Input: part model. Units: mm. Frame: model coordinates. Face numbers are marked on the shaded views. A direction names the side the tool comes from. Round coordinates to 2 decimals unless told otherwise and drop trailing zeros. Write each loop counter-clockwise with the first axis right and the second up, starting at its lowest first coordinate (ties: lowest second). Pieces come first, ordered by that corner, then holes. Notation, with made-up numbers: M -28,-8.75 L -20,-8.75 A21 cw -20,26.25 Z; hole C 40.5,12 d5. An arc over 180 degrees is marked long. Answer as CSV lines item,"result". Start each with the question number.
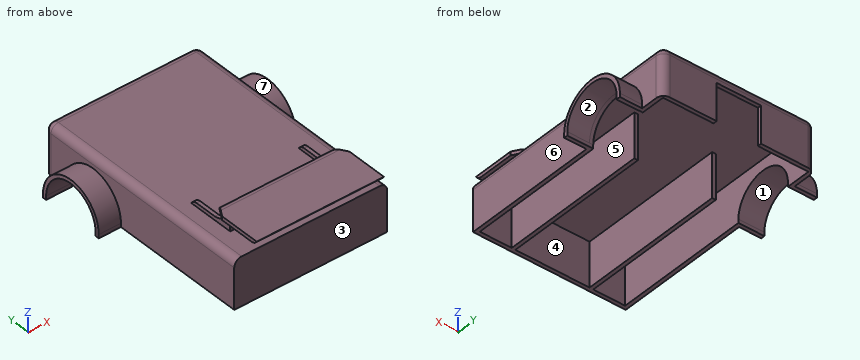
```python
from build123d import *

# Parameters (mm, degrees)
SKETCH1_W               = 206
SKETCH1_H               = 306
BOSS_EXTRUDE2_DEPTH     = 5
SKETCH2_W               = 206
SKETCH2_H               = 306
SKETCH2_W_2             = 196
SKETCH2_H_2             = 296
BOSS_EXTRUDE3_DEPTH     = 60
SKETCH3_W               = 5
SKETCH3_H               = 198
BOSS_EXTRUDE4_DEPTH     = 60
SKETCH10_W              = 60
SKETCH10_H              = 5
CUT_EXTRUDE3_DEPTH      = 50
CUT_EXTRUDE4_DEPTH      = 296.372645991
CUT_EXTRUDE4_DEPTH_BACK = 5
BOSS_EXTRUDE6_DEPTH     = 30
CUT_EXTRUDE5_DEPTH      = 318.025235589
CUT_EXTRUDE5_DEPTH_BACK = 5
BOSS_EXTRUDE7_DEPTH     = 30
SKETCH16_W              = 5
SKETCH16_H              = 63
BOSS_EXTRUDE8_DEPTH     = 5
BOSS_EXTRUDE10_DEPTH    = 150
SKETCH19_W              = 140
SKETCH19_H              = 20
CUT_EXTRUDE6_DEPTH      = 70
BOSS_EXTRUDE11_DEPTH    = 5
FILLET3_R               = 10
FILLET4_R               = 10
FILLET5_R               = 10
FILLET6_R               = 10
FILLET7_R               = 10
FILLET8_R               = 10
FILLET9_R               = 10


with BuildPart() as part:
    # Sketch1 → Boss-Extrude2 (new body)
    with BuildSketch(Plane.XY):
        with Locations((0, 50)):
            Rectangle(SKETCH1_W, SKETCH1_H)
    extrude(amount=BOSS_EXTRUDE2_DEPTH)

    # Sketch2 → Boss-Extrude3 (add)
    with BuildSketch(Plane(origin=(0, 0, 0), x_dir=(-1, 0, 0), z_dir=(0, 0, -1))):
        with Locations((0, 50)):
            Rectangle(SKETCH2_W, SKETCH2_H)
        with Locations((0, 50)):
            Rectangle(SKETCH2_W_2, SKETCH2_H_2, mode=Mode.SUBTRACT)
    extrude(amount=BOSS_EXTRUDE3_DEPTH)

    # Sketch3 → Boss-Extrude4 (add)
    with BuildSketch(Plane(origin=(0, 0, 0), x_dir=(-1, 0, 0), z_dir=(0, 0, -1))):
        with Locations((-52.5, 1)):
            Rectangle(SKETCH3_W, SKETCH3_H)
        with Locations((52.5, 1)):
            Rectangle(SKETCH3_W, SKETCH3_H)
    extrude(amount=BOSS_EXTRUDE4_DEPTH)

    # Sketch10 → Cut-Extrude3 (cut)
    with BuildSketch(Plane(origin=(0, 0, -60), x_dir=(-1, 0, 0), z_dir=(0, 0, -1))):
        with Locations((0, 200.5)):
            Rectangle(SKETCH10_W, SKETCH10_H)
    extrude(amount=-CUT_EXTRUDE3_DEPTH, mode=Mode.SUBTRACT)

    # Sketch11 → Cut-Extrude4 (cut, two sides: drawn at the far end of the back side and taken through both)
    with BuildSketch(Plane(origin=(103, 0, 0), x_dir=(0, 0, -1), z_dir=(1, 0, 0)).offset(-CUT_EXTRUDE4_DEPTH_BACK)):
        with BuildLine():
            Line((55, 165.246993189), (60, 165.246993189))
            Line((60, 165.246993189), (60, 85.246993189))
            Line((60, 85.246993189), (55, 85.246993189))
            ThreePointArc((55, 85.246993189), (15, 125.246993189), (55, 165.246993189))
        make_face()
    extrude(amount=CUT_EXTRUDE4_DEPTH + CUT_EXTRUDE4_DEPTH_BACK, mode=Mode.SUBTRACT)

    # Sketch12 → Boss-Extrude6 (add)
    with BuildSketch(Plane(origin=(103, 0, 0), x_dir=(0, 0, -1), z_dir=(1, 0, 0))):
        with BuildLine():
            Line((55, 170.246993189), (60, 170.246993189))
            Line((60, 170.246993189), (60, 164.922358247))
            Line((60, 164.922358247), (55, 164.922358247))
            ThreePointArc((55, 164.922358247), (15.162317471, 125.084675718), (55, 85.246993189))
            Line((55, 85.246993189), (60, 85.246993189))
            Line((60, 85.246993189), (60, 80.246993189))
            Line((60, 80.246993189), (55, 80.246993189))
            ThreePointArc((55, 80.246993189), (10, 125.246993189), (55, 170.246993189))
        make_face()
    extrude(amount=BOSS_EXTRUDE6_DEPTH)

    # Sketch13 → Cut-Extrude5 (cut, two sides: drawn at the far end of the back side and taken through both)
    with BuildSketch(Plane.ZY.offset(103).offset(-CUT_EXTRUDE5_DEPTH_BACK)):
        with BuildLine():
            Line((-55, 165), (-60, 165))
            Line((-60, 165), (-60, 85))
            Line((-60, 85), (-55, 85))
            ThreePointArc((-55, 85), (-15, 125), (-55, 165))
        make_face()
    extrude(amount=CUT_EXTRUDE5_DEPTH + CUT_EXTRUDE5_DEPTH_BACK, mode=Mode.SUBTRACT)

    # Sketch14 → Boss-Extrude7 (add)
    with BuildSketch(Plane.ZY.offset(103)):
        with BuildLine():
            Line((-55, 170), (-60, 170))
            Line((-60, 170), (-60, 165))
            Line((-60, 165), (-55, 165))
            ThreePointArc((-55, 165), (-15, 125), (-55, 85))
            Line((-55, 85), (-60, 85))
            Line((-60, 85), (-60, 80))
            Line((-60, 80), (-55, 80))
            ThreePointArc((-55, 80), (-10, 125), (-55, 170))
        make_face()
    extrude(amount=BOSS_EXTRUDE7_DEPTH)

    # Sketch16 → Boss-Extrude8 (add)
    with BuildSketch(Plane.XY.offset(5)):
        with Locations((-72.5, -31.5)):
            Rectangle(SKETCH16_W, SKETCH16_H)
        with Locations((72.5, -31.5)):
            Rectangle(SKETCH16_W, SKETCH16_H)
    extrude(amount=BOSS_EXTRUDE8_DEPTH)

    # Sketch17 → Boss-Extrude10 (add)
    with BuildSketch(Plane.ZY.offset(75)):
        with BuildLine():
            Line((5, -63), (30, -63))
            Line((30, -63), (30, -57.184020249))
            ThreePointArc((30, -57.184020249), (16.143353283, -51.612696786), (10, -38))
            Line((10, -38), (10, 0))
            Line((10, 0), (5, 0))
            Line((5, 0), (5, -63))
        make_face()
    extrude(amount=-BOSS_EXTRUDE10_DEPTH)

    # Sketch19 → Cut-Extrude6 (cut)
    with BuildSketch(Plane.XZ.offset(63)):
        with Locations((0, 15)):
            Rectangle(SKETCH19_W, SKETCH19_H)
    extrude(amount=-CUT_EXTRUDE6_DEPTH, mode=Mode.SUBTRACT)

    # Sketch20 → Boss-Extrude11 (add)
    with BuildSketch(Plane.XY.offset(30)):
        Polygon((75, -45.439640401), (-75, -45.439640401), (-85.792774028, -63), (-85.792774028, -118.716663175), (85.792774028, -118.716663175), (85.792774028, -63), align=None)
    extrude(amount=-BOSS_EXTRUDE11_DEPTH)

    # Fillet3
    fillet3_edges = [part.edges().sort_by_distance(p)[0] for p in [
        (-103, 203, -27.5),
    ]]
    fillet(fillet3_edges, radius=FILLET3_R)

    # Fillet4
    fillet4_edges = [part.edges().sort_by_distance(p)[0] for p in [
        (103, 203, -27.5),
    ]]
    fillet(fillet4_edges, radius=FILLET4_R)

    # Fillet5
    # the kernel refuses this fillet: 10 mm, written as the material it takes off along each edge
    with BuildSketch(Plane(origin=(96.650635095, -45.439640401, 30), x_dir=(0, 0, -1), z_dir=(-1, 0, 0))) as fillet5_piece_1:
        with BuildLine():
            CenterArc((10, 8.660254038), FILLET5_R, 180, 60)
            Line((0, 8.660254038), (-0.2, 8.660254038))
            Line((-0.2, 8.660254038), (-0.2, 0))
            Line((-0.2, 0), (0, -0.2))
            ThreePointArc((0, -0.2), (2.5, -0.2), (4.9, -0.173205081))
            Line((4.9, -0.173205081), (5, 0))
        make_face()
    extrude(amount=193.301270189, mode=Mode.SUBTRACT)

    # Fillet6
    # the kernel refuses this fillet: 10 mm, written as the material it takes off along each edge
    with BuildSketch(Plane(origin=(-107.443409123, -118.716663175, 25), x_dir=(0, 1, 0), z_dir=(1, 0, 0))) as fillet6_piece_1:
        with BuildLine():
            CenterArc((8.660254038, 10), FILLET6_R, 210, 60)
            Line((0, 5), (-0.173205081, 4.9))
            ThreePointArc((-0.173205081, 4.9), (-0.2, 2.5), (-0.2, 0))
            Line((-0.2, 0), (0, -0.2))
            Line((0, -0.2), (8.660254038, -0.2))
            Line((8.660254038, -0.2), (8.660254038, 0))
        make_face()
    extrude(amount=214.886818246, mode=Mode.SUBTRACT)

    # Fillet7
    # the kernel refuses this fillet: 10 mm, written as the material it takes off along each edge
    with BuildSketch(Plane(origin=(-96.650635095, 0, 10), x_dir=(0, 0, -1), z_dir=(1, 0, 0))) as fillet7_piece_1:
        with BuildLine():
            CenterArc((10, -8.660254038), FILLET7_R, 120, 60)
            Line((0, -8.660254038), (-0.2, -8.660254038))
            Line((-0.2, -8.660254038), (-0.2, 0))
            Line((-0.2, 0), (0, 0.2))
            ThreePointArc((0, 0.2), (2.5, 0.2), (4.9, 0.173205081))
            Line((4.9, 0.173205081), (5, 0))
        make_face()
    extrude(amount=48.301270189, mode=Mode.SUBTRACT)

    # Fillet8
    # the kernel refuses this fillet: 10 mm, written as the material it takes off along each edge
    with BuildSketch(Plane(origin=(48.349364905, 0, 10), x_dir=(0, 0, -1), z_dir=(1, 0, 0))) as fillet8_piece_1:
        with BuildLine():
            CenterArc((10, -8.660254038), FILLET8_R, 120, 60)
            Line((0, -8.660254038), (-0.2, -8.660254038))
            Line((-0.2, -8.660254038), (-0.2, 0))
            Line((-0.2, 0), (0, 0.2))
            ThreePointArc((0, 0.2), (2.5, 0.2), (4.9, 0.173205081))
            Line((4.9, 0.173205081), (5, 0))
        make_face()
    extrude(amount=48.301270189, mode=Mode.SUBTRACT)

    # Fillet9
    # the kernel refuses this fillet: 10 mm, written as the material it takes off along each edge
    with BuildSketch(Plane(origin=(103, 193, 5), x_dir=(-1, 0, 0), z_dir=(0, -1, 0)), Plane(origin=(-103, -128, 5), x_dir=(1, 0, 0), z_dir=(0, 1, 0))) as fillet9_piece_1:
        with BuildLine():
            CenterArc((FILLET9_R, FILLET9_R), FILLET9_R, 180, 90)
            Line((0, FILLET9_R), (0, 0))
            Line((0, 0), (FILLET9_R, 0))
        make_face()
    extrude(amount=321, mode=Mode.SUBTRACT)
    with BuildSketch(Plane(origin=(-93, 193, 5), x_dir=(-1, 0, 0), z_dir=(0, -1, 0))) as fillet9_piece_2:
        with BuildLine():
            CenterArc((10 - FILLET9_R, FILLET9_R), FILLET9_R, 270, 90)
            Line((10, FILLET9_R), (10, 0))
            Line((10, 0), (10 - FILLET9_R, 0))
        make_face()
    revolve(axis=Axis((-93, 193, 5), (0, 0, -1)), revolution_arc=90, mode=Mode.SUBTRACT)
    with BuildSketch(Plane(origin=(-93, 203, 5), x_dir=(0, -1, 0), z_dir=(1, 0, 0))) as fillet9_piece_3:
        with BuildLine():
            CenterArc((FILLET9_R, FILLET9_R), FILLET9_R, 180, 90)
            Line((0, FILLET9_R), (0, 0))
            Line((0, 0), (FILLET9_R, 0))
        make_face()
    extrude(amount=186, mode=Mode.SUBTRACT)
    with BuildSketch(Plane(origin=(93, 193, 5), x_dir=(0, 1, 0), z_dir=(-1, 0, 0))) as fillet9_piece_4:
        with BuildLine():
            CenterArc((10 - FILLET9_R, FILLET9_R), FILLET9_R, 270, 90)
            Line((10, FILLET9_R), (10, 0))
            Line((10, 0), (10 - FILLET9_R, 0))
        make_face()
    revolve(axis=Axis((93, 193, 5), (0, 0, -1)), revolution_arc=90, mode=Mode.SUBTRACT)


solid = part.part
```
Item 1: Cut plane B-B, the plane y = 52.5. Return loops of the section in (x, z).
Item 2: Cut plane A-A, the plane x = 64. Return loops of the section in (y, z), plus the area to 3 significant figures.
Item 3: Access query for the marked faces 1, 2, 3 and 4. Directions: +Z, -Z, +X, -X, +Y, -Y. A direction counts if a zero-diameter tool reaches every point of the face in a straight line with its end or side. Return the directions, or none.
Item 4: Draft query along Y for the marked faces 5, 6 and 7. Return one class per face: +Y half, -Y half, draft (parallel to the pull), parting line (faces both ways), or undercut.
Item 5: Pin query (flat end, axial travel): pin 1 Ø4 at (x, z) = (-110, -57.5) entering from +Y; pin 2 Ø1.5 at (x, z) = (109, -57) entering from +Y; pin 3 Ø16 at (y, z) = (-26.5, 10.5) entering from -X. Return the tip coordinate at first contact, or that it passes through.
Item 6: Line query: line 1 (X direction, y = 59, z = -52); line 2 (X direction, y = 92, z = -46); line 3 (X direction, y = 149, z = -20). Output: solid intervals per line, ascending. Write a range as [from, to].
Item 7: Cut plane C-C, the plane y = 90.5. Return loops of the section in (x, z).
Item 8: Cut plane D-D, the plane z = -43. Give the number of separate pieces and of enclosed holes in the cut face, plus the area to 3 significant figures.
Results list:
1,outline,"M -103,-60 L -98,-60 L -98,0 L -55,0 L -55,-60 L -50,-60 L -50,0 L 50,0 L 50,-60 L 55,-60 L 55,0 L 98,0 L 98,-60 L 103,-60 L 103,-5 A10 ccw 93,5 L -93,5 A10 ccw -103,-5 Z"
2,outline,"M -118.72,30 A10 ccw -110.06,25 L -45.44,25 A10 ccw -54.1,30 Z; M -103,-60 L -98,-60 L -98,0 L 198,0 L 198,-60 L 203,-60 L 203,-5 A10 ccw 193,5 L -103,5 Z"
2,area,"2,450 mm²"
3,face 1,"-Z, -X"
3,face 2,"-Z, +X"
3,face 3,"-Z, +X, -X, -Y"
3,face 4,"-Z"
4,face 5,"undercut"
4,face 6,"draft"
4,face 7,"parting line"
5,pin 1,"y = 170"
5,pin 2,"y = 170.25"
5,pin 3,"x = -99.61"
6,line 1,"[-103, -98], [-55, -50], [50, 55], [98, 103]"
6,line 2,"[-55, -50], [50, 55]"
6,line 3,"[-133, -98], [98, 133]"
7,outline,"M -133,-34.76 L -98,-34.76 L -98,0 L -55,0 L -55,-60 L -50,-60 L -50,0 L 50,0 L 50,-60 L 55,-60 L 55,0 L 98,0 L 98,-35.18 L 103,-35.18 L 103,-35.23 L 133,-35.23 L 133,-26.41 L 103,-26.41 L 103,-5 A10 ccw 93,5 L -93,5 A10 ccw -103,-5 L -103,-26.11 L -133,-26.11 Z"
8,separate pieces,"3"
8,enclosed holes,"0"
8,area,"6,530 mm²"
